Part model, mm, in its own coordinate system. A direction names the side the tool comes from. Coordinates: 2 decimals unless noted, no trailing zeros. Write each loop counter-clockwise with the first axis right and the second up, starting at its lowest first coordinate (ties: lowest second). Pieces come first, ordered by that corner, then holes. Notation, with made-up numbers: (-25, 52) - (1, 52) arc R16 ccw to (1, 63) - close; hole circle Ø9 at (57.5, -23). An arc over 180 degrees is marked (long way). Use one line per item in the form item = value. Start each with the question number.
from build123d import *

# Parameters (mm, degrees)
F1_DEPTH       = 3
F2_R           = 3.5
F3_DEPTH       = 4
F5_D           = 4.5
F5_CSINK_D     = 9
F5_CSINK_ANGLE = 90
F6_R           = 1.5


# Not quite as in the source:
# - a feature names something its author has since deleted; it is built from what else it names


with BuildPart() as f1:
    # F0 (on Top) → F1 (new body)
    with BuildSketch(Plane.XY):
        with BuildLine():
            ThreePointArc((6, 12.5), (0, 18.5), (-6, 12.5))
            Line((-6, 12.5), (-6, -12.5))
            ThreePointArc((-6, -12.5), (0, -18.5), (6, -12.5))
            Line((6, -12.5), (6, 12.5))
        make_face()
    extrude(amount=F1_DEPTH)

    # F2 (on face) → F3 (join)
    with BuildSketch(Plane.XY.offset(3)):
        with Locations((0, -12.5)):
            Circle(F2_R)
        with Locations((0, 12.5)):
            Circle(F2_R)
    extrude(amount=F3_DEPTH)

    # F5 (through all)
    with Locations(Plane(origin=(0, 0, 0), x_dir=(1, 0, 0), z_dir=(0, 0, -1))):
        with Locations((0, 12.5), (0, -12.5)):
            CounterSinkHole(F5_D / 2, F5_CSINK_D / 2, counter_sink_angle=F5_CSINK_ANGLE)

    # F6
    f6_edges = [f1.edges().sort_by_distance(p)[0] for p in [
        (-6, 0, 3),
    ]]
    fillet(f6_edges, radius=F6_R)


solid = f1.part
Q1. Pin check, flat tips, straight feed: P1, Ø3, axis at y = -12, z = 6, coming from the +X side; P2, Ø1, axis at x = -1.5, z = 3, coming from the -Y side; P3, Ø2.5, axis at x = 0, y = 12.5, coming from the +Z side. Stop position of each tip, or through.
Q2. Slice it at C-C (y = 2.5). List the corners of the cut face in (x, z).
Q3. Drill centre lines: probe 1 along Y at (x, z) = (0, 4.6); probe 2 along Y at (x, z) = (-1, 3.75); probe 3 along Z at (x, y) = (-1, -6). Where is each one in solid material? Low to high.
Q4. Mould opens along X. For faces 1 (the cylindrical face through (0.29, -14.73, 4.66)), 2 (the cylindrical face through (-5.55, -0.18, 2.57)), 3 (the cylindrical face through (5.55, 0.18, 2.57)) say: released by +X, released by -X, zero draft, split by the parting line, or undercut.
Q5. Slice it at B-B (z = 5). List the corners of the cut face in (x, y).
Q6. Which spindle directions (+Z, -Z, +X, -X, +Y, -Y) get a long thin tool onto all of the face, cutting with end or side? Do faces 4 (the flat face through (-6, 0, 1)), 5 (the cylindrical face through (-0.759, 9.083, 4.972)). Say none if no direction does.
Q7. Slice it at A-A (x = 0). List the corners of the cut face in (y, z).
Solution:
q1.P1 = 3.5
q1.P2 = -17.93
q1.P3 = through
q2.outline = (-6, 0) - (6, 0) - (6, 1.5) arc R1.5 ccw to (4.5, 3) - (-4.5, 3) arc R1.5 ccw to (-6, 1.5) - close
q3.probe_1 = -16 to -14.75, -10.25 to -9, 9 to 10.25, 14.75 to 16
q3.probe_2 = -15.85 to -14.52, -10.48 to -9.15, 9.15 to 10.48, 14.52 to 15.85
q3.probe_3 = 0 to 3
q4.face_1 = undercut
q4.face_2 = released by -X
q4.face_3 = released by +X
q5.outline = circle Ø7 at (0, -12.5); circle Ø7 at (0, 12.5); hole circle Ø4.5 at (0, -12.5); hole circle Ø4.5 at (0, 12.5)
q6.face_4 = +Z, -Z, -X, +Y, -Y
q6.face_5 = +Z
q7.outline = (-18.5, 0) - (-17, 0) - (-14.75, 2.25) - (-14.75, 7) - (-16, 7) - (-16, 3) - (-17, 3) arc R1.5 ccw to (-18.5, 1.5) - close; (-10.25, 2.25) - (-8, 0) - (8, 0) - (10.25, 2.25) - (10.25, 7) - (9, 7) - (9, 3) - (-9, 3) - (-9, 7) - (-10.25, 7) - close; (14.75, 2.25) - (17, 0) - (18.5, 0) - (18.5, 1.5) arc R1.5 ccw to (17, 3) - (16, 3) - (16, 7) - (14.75, 7) - close
